from build123d import *

# Parameters (mm, degrees)
BOSS_EXTRU_1_DEPTH                              = 8
CONG_1_R                                        = 0.5
ESQUISSE6_R                                     = 1.6
ENL_V_MAT_EXTRU_1_DEPTH                         = 10.5
ESQUISSE7_W                                     = 5.85
ESQUISSE7_H                                     = 2.25
ENL_V_MAT_EXTRU_2_DEPTH                         = 9.0000001
BOSS_EXTRU_2_DEPTH                              = 3
CHAMBRAGE_POUR_VIS_T_TE_CYLINDRIQUE_D           = 2.5
CHAMBRAGE_POUR_VIS_T_TE_CYLINDRIQUE_CBORE_D     = 4.5
CHAMBRAGE_POUR_VIS_T_TE_CYLINDRIQUE_CBORE_DEPTH = 5.3
ESQUISSE14_R                                    = 4.25
ENL_V_MAT_EXTRU_3_DEPTH                         = 2


with BuildPart() as part:
    # Esquisse1 → Boss.-Extru.1 (new body)
    with BuildSketch(Plane(origin=(0, 0, 0), x_dir=(1, 0, 0), z_dir=(0, 1, 0))):
        with BuildLine():
            Line((6.025985397, 9.5), (-6.025985397, 9.5))
            ThreePointArc((-6.025985397, 9.5), (0, -11.25), (6.025985397, 9.5))
        make_face()
        with BuildLine():
            Line((-3.2, 0), (-3.2, 2.9))
            Line((-3.2, 2.9), (3.2, 2.9))
            Line((3.2, 2.9), (3.2, 0))
            ThreePointArc((3.2, 0), (0, -3.2), (-3.2, 0))
        make_face(mode=Mode.SUBTRACT)
    extrude(amount=BOSS_EXTRU_1_DEPTH)

    # Congé1
    cong_1_edges = [part.edges().sort_by_distance(p)[0] for p in [
        (0, 8, 3.2),
        (3.2, 8, -1.45),
        (0, 8, -2.9),
        (-3.2, 8, -1.45),
    ]]
    fillet(cong_1_edges, radius=CONG_1_R)

    # Esquisse6 → Enlèv. mat.-Extru.1 (cut, through all)
    with BuildSketch(Plane.XY):
        with Locations((0, 4)):
            Circle(ESQUISSE6_R)
    extrude(amount=-ENL_V_MAT_EXTRU_1_DEPTH, mode=Mode.SUBTRACT)

    # Esquisse7 → Enlèv. mat.-Extru.2 (cut, through all)
    with BuildSketch(Plane(origin=(0, 0, 0), x_dir=(1, 0, 0), z_dir=(0, 1, 0))):
        with Locations((0, 5.525)):
            Rectangle(ESQUISSE7_W, ESQUISSE7_H)
    extrude(amount=ENL_V_MAT_EXTRU_2_DEPTH, mode=Mode.SUBTRACT)

    # Esquisse8 → Boss.-Extru.2 (add)
    with BuildSketch(Plane.XZ):
        with BuildLine():
            Line((-6.025985397, -9.5), (6.025985397, -9.5))
            ThreePointArc((6.025985397, -9.5), (0, 11.25), (-6.025985397, -9.5))
        make_face()
    extrude(amount=BOSS_EXTRU_2_DEPTH)

    # Chambrage pour vis à tête cylindrique à 6 pans creux (ou vis CHC) M21 (through all)
    with Locations(Plane(origin=(0, 8, 0), x_dir=(1, 0, 0), z_dir=(0, 1, 0))):
        with Locations((-8, 0), (0, -8), (8, 0)):
            CounterBoreHole(CHAMBRAGE_POUR_VIS_T_TE_CYLINDRIQUE_D / 2, CHAMBRAGE_POUR_VIS_T_TE_CYLINDRIQUE_CBORE_D / 2, CHAMBRAGE_POUR_VIS_T_TE_CYLINDRIQUE_CBORE_DEPTH)

    # Esquisse14 → Enlèv. mat.-Extru.3 (cut)
    with BuildSketch(Plane.XZ.offset(3)):
        Circle(ESQUISSE14_R)
    extrude(amount=-ENL_V_MAT_EXTRU_3_DEPTH, mode=Mode.SUBTRACT)


solid = part.part
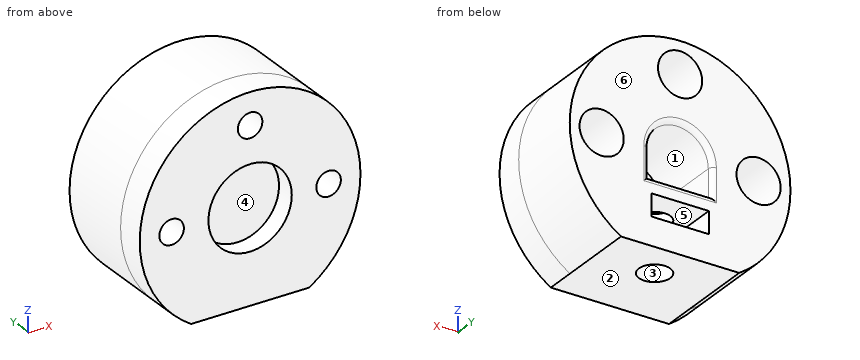
Could you check a few things on this model? Use its own coordinates, in mm. Face numbers are marked on the shaded views. A direction names the side the tool comes from. Give positions to 0.01 mm unless a question says otherwise; leave off trailing zeros. Order: outer loops, then holes, each group sorted by start corner. A loop starts at its lowest first (then second) coordinate and runs counter-clockwise, first axis right, second up. Notation, with made-up numbers: M 53,11.25 L 107,11.25 A14 cw 107,38.25 Z; hole C 27,-28 d4. An arc over 180 degrees is marked long. One line per question, with ' | ' between items.
1. I want a section at A-A (y = 6.5). List the corners of the cut face in (x, z) for me (3 decimals).
Results:
outline: M -6.026,-9.5 L 6.026,-9.5 A11.25 ccw long Z; hole C -8,0 d4.5; hole M -3.2,-2.9 L 3.2,-2.9 L 3.2,0 A3.2 ccw -3.2,0 Z; hole M -2.925,-6.65 L 2.925,-6.65 L 2.925,-4.4 L -2.925,-4.4 Z; hole C 0,8 d4.5; hole C 8,0 d4.5
2. We'd pull the mould along Z, two halves only. Please class the marked faces 1, 2 and 3: +Z half, -Z half, draft (parallel to the pull), parting line (faces both ways), or undercut.
Results:
face 1: undercut | face 2: -Z half | face 3: draft
3. I want a section at C-C (z = 8). List the corners of the cut face in (x, y) for me.
Results:
outline: M -7.91,-3 L -1.25,-3 L -1.25,2.7 L -2.25,2.7 L -2.25,8 L -7.91,8 Z; M 1.25,-3 L 7.91,-3 L 7.91,8 L 2.25,8 L 2.25,2.7 L 1.25,2.7 Z
4. If I drill on line 1 (Z direction, x = 0, y = -2.5); line 2 (X direction, y = -1.5, z = 1); line 3 (X direction, y = 0.5, z = 1), over which ranges is the centre line in solid material (lowest first)?
Results:
line 1: -9.5 to -4.25, 4.25 to 6.75, 9.25 to 11.25 | line 2: -11.21 to -8.75, -7.25 to -4.13, 4.13 to 7.25, 8.75 to 11.21 | line 3: -11.21 to -8.75, -7.25 to -3.04, 3.04 to 7.25, 8.75 to 11.21
5. For the marked faces 4, 5 and 6, which set-ups out of +Z, -Z, +X, -X, +Y, -Y let a thin tool reach every point of the face, with its end or its side?
Results:
face 4: -Y | face 5: +Y | face 6: +Z, -Z, +X, -X, +Y
6. I want a section at D-D (y = 4). List the corners of the cut face in (x, z) for me (3 decimals), and give its area (3 significant figures).
Results:
outline: M -6.026,-9.5 L -1.6,-9.5 L -1.6,-6.65 L -2.925,-6.65 L -2.925,-4.4 L -1.6,-4.4 L -1.6,-2.9 L -3.2,-2.9 L -3.2,0 A3.2 cw 3.2,0 L 3.2,-2.9 L 1.6,-2.9 L 1.6,-4.4 L 2.925,-4.4 L 2.925,-6.65 L 1.6,-6.65 L 1.6,-9.5 L 6.026,-9.5 A11.25 ccw long Z; hole C -8,0 d4.5; hole C 0,8 d4.5; hole C 8,0 d4.5 | area: 274 mm²
7. I'm going to push flat-ended pins straight in: pin 1 (2.5 mm diameter, centred on y = 4.5, z = -5.5, fed in from +X); pin 2 (1.8 mm diameter, centred on x = 0.5, z = -5.5, fed in from +Y); pin 3 (0.7 mm diameter, centred on y = 3, z = -5.5, fed in from -X). Where does each tip first touch, or does it pass through?
Results:
pin 1: x = 10.42 | pin 2: y = 0 | pin 3: x = -10
8. I want a section at B-B (x = -8). List the corners of the cut face in (y, z) for me.
Results:
outline: M -3,-7.91 L 8,-7.91 L 8,-2.25 L 2.7,-2.25 L 2.7,-1.25 L -3,-1.25 Z; M -3,1.25 L 2.7,1.25 L 2.7,2.25 L 8,2.25 L 8,7.91 L -3,7.91 Z
